Geometry check sheet. Reference: the model listing, model coordinates, mm. Coordinates: 2 decimals unless noted, no trailing zeros. Order: outer loops, then holes, each group sorted by start corner. A loop starts at its lowest first (then second) coordinate and runs counter-clockwise, first axis right, second up. Notation, with made-up numbers: (-5, 57.5) -> (22, 57.5) arc R28 cw to (22, 94.5) -> close; hole circle Ø4 at (78, 7). An arc over 180 degrees is marked (long way). Answer as CSV lines item,"result". Start each with the question number.
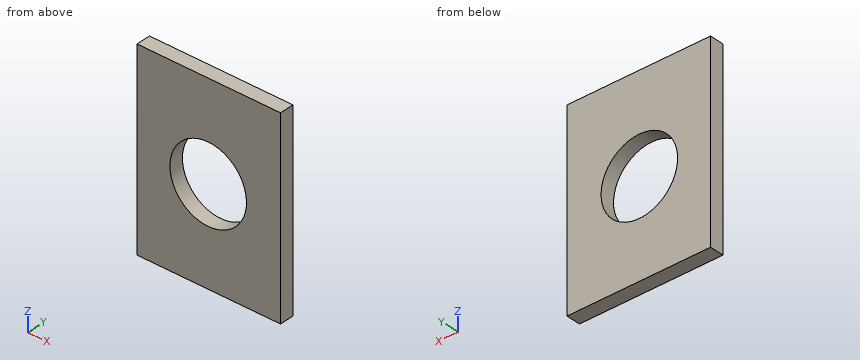
from build123d import *

# Parameters (mm, degrees)
BOSS_EXTRUDE1_DEPTH = 20
BOSS_EXTRUDE2_DEPTH = 1.5
SKETCH3_W           = 10
SKETCH3_H           = 2
BOSS_EXTRUDE3_DEPTH = 100
SKETCH4_R           = 1.55
CUT_EXTRUDE1_DEPTH  = 2
SKETCH5_R           = 4
CUT_EXTRUDE2_DEPTH  = 3
CUT_EXTRUDE3_START  = -2
CUT_EXTRUDE3_DEPTH  = 2
SKETCH7_W           = 92.843167551
SKETCH7_H           = 36.119357845
CUT_EXTRUDE4_DEPTH  = 30
SKETCH8_W           = 90.626752411
SKETCH8_H           = 35.380552798
CUT_EXTRUDE5_DEPTH  = 55
SKETCH10_W          = 29.390209747
SKETCH10_H          = 30.061690813
CUT_EXTRUDE7_DEPTH  = 20
SKETCH11_W          = 23.008025921
SKETCH11_H          = 26.899718038
CUT_EXTRUDE8_DEPTH  = 40


# Read off the part's stored shape, not the designer's step: Boss-Extrude1, Cut-Extrude3
with BuildPart() as part:
    # Boss-Extrude1 outline → Boss-Extrude1 (new body)
    with BuildSketch(Plane(origin=(0, 0, 0), x_dir=(1, 0, 0), z_dir=(0, 1, 0))):
        with BuildLine():
            Line((49.999999852, 30), (4.999999852, 30))
            ThreePointArc((4.999999852, 30), (1.464465946, 31.464466094), (-1.48e-07, 35))
            Line((-1.48e-07, 35), (-1.48e-07, 40))
            Line((-1.48e-07, 40), (-40.000000148, 40))
            Line((-40.000000148, 40), (-40.000000111, 35))
            ThreePointArc((-40.000000111, 35), (-41.464466194, 31.46446612), (-45.000000074, 30.000000037))
            Line((-45.000000074, 30.000000037), (-50.000000148, 30))
            Line((-50.000000148, 30), (-50.000000148, -30))
            Line((-50.000000148, -30), (49.999999852, -30))
            Line((49.999999852, -30), (49.999999852, 30))
        make_face()
        with BuildLine():
            Line((-48.5, 28.5), (-44.999018222, 28.5))
            ThreePointArc((-44.999018222, 28.5), (-40.40345882, 30.40415302), (-38.5, 35))
            Line((-38.5, 35), (-38.5, 38.5))
            Line((-38.5, 38.5), (-1.500000148, 38.5))
            Line((-1.500000148, 38.5), (-1.500000148, 35))
            ThreePointArc((-1.500000148, 35), (0.403805774, 30.403805922), (4.999999852, 28.5))
            Line((4.999999852, 28.5), (48.5, 28.5))
            Line((48.5, 28.5), (48.5, -28.5))
            Line((48.5, -28.5), (-48.5, -28.5))
            Line((-48.5, -28.5), (-48.5, 28.5))
        make_face(mode=Mode.SUBTRACT)
    extrude(amount=BOSS_EXTRUDE1_DEPTH)

    # Sketch2 → Boss-Extrude2 (add)
    with BuildSketch(Plane(origin=(0, 20, 0), x_dir=(1, 0, 0), z_dir=(0, 1, 0))):
        with BuildLine():
            Line((-40.000000148, 40), (-1.48e-07, 40))
            Line((-1.48e-07, 40), (-1.48e-07, 35))
            ThreePointArc((-1.48e-07, 35), (1.464465946, 31.464466094), (4.999999852, 30))
            Line((4.999999852, 30), (49.999999852, 30))
            Line((49.999999852, 30), (49.999999852, -30))
            Line((49.999999852, -30), (-50.000000148, -30))
            Line((-50.000000148, -30), (-50.000000148, 30))
            Line((-50.000000148, 30), (-45.000000074, 30))
            ThreePointArc((-45.000000074, 30), (-41.464466216, 31.46446612), (-40.000000148, 35))
            Line((-40.000000148, 35), (-40.000000148, 40))
        make_face()
    extrude(amount=BOSS_EXTRUDE2_DEPTH)

    # Sketch3 → Boss-Extrude3 (add)
    with BuildSketch(Plane(origin=(49.999999852, 0, 0), x_dir=(0, 0, -1), z_dir=(1, 0, 0))):
        with Locations((35, 1)):
            Rectangle(SKETCH3_W, SKETCH3_H)
        with Locations((-35, 1)):
            Rectangle(SKETCH3_W, SKETCH3_H)
    extrude(amount=-BOSS_EXTRUDE3_DEPTH)

    # Sketch4 → Cut-Extrude1 (cut)
    with BuildSketch(Plane.XZ):
        with Locations(Location((-45, 35, 0), (0, 0, 270))):
            Circle(SKETCH4_R)
        with Locations(Location((45, 35, 0), (0, 0, 270))):
            Circle(SKETCH4_R)
        with Locations(Location((45, -35, 0), (0, 0, 270))):
            Circle(SKETCH4_R)
        with Locations(Location((-45, -35, 0), (0, 0, 270))):
            Circle(SKETCH4_R)
        with Locations(Location((5, 35, 0), (0, 0, 270))):
            Circle(SKETCH4_R)
        with Locations(Location((5, -35, 0), (0, 0, 270))):
            Circle(SKETCH4_R)
    extrude(amount=-CUT_EXTRUDE1_DEPTH, mode=Mode.SUBTRACT)

    # Sketch5 → Cut-Extrude2 (cut)
    with BuildSketch(Plane(origin=(0, 21.5, 0), x_dir=(1, 0, 0), z_dir=(0, 1, 0))):
        with Locations(Location((12.44, -9.95, 0), (0, 0, 270))):
            Circle(SKETCH5_R)
    extrude(amount=-CUT_EXTRUDE2_DEPTH, mode=Mode.SUBTRACT)

    # Cut-Extrude3 outline → Cut-Extrude3 (cut)
    with BuildSketch(Plane(origin=(0, 2, 0), x_dir=(1, 0, 0), z_dir=(0, 1, 0)).offset(CUT_EXTRUDE3_START)):
        with BuildLine():
            Line((-38.5, 38.5), (-38.5, 35))
            ThreePointArc((-38.5, 35), (-39.115846372, 32.238345392), (-40.846688027, 30))
            Line((-40.846688027, 30), (0.84668792, 30))
            ThreePointArc((0.84668792, 30), (-0.884153764, 32.238345383), (-1.500000148, 35))
            Line((-1.500000148, 35), (-1.500000148, 38.5))
            Line((-1.500000148, 38.5), (-38.5, 38.5))
        make_face()
    extrude(amount=CUT_EXTRUDE3_DEPTH, mode=Mode.SUBTRACT)

    # Sketch7 → Cut-Extrude4 (cut)
    with BuildSketch(Plane(origin=(49.999999852, 0, 0), x_dir=(0, 0, -1), z_dir=(1, 0, 0))):
        with Locations((0.287313074, 10.115071794)):
            Rectangle(SKETCH7_W, SKETCH7_H)
    extrude(amount=-CUT_EXTRUDE4_DEPTH, mode=Mode.SUBTRACT)

    # Sketch8 → Cut-Extrude5 (cut)
    with BuildSketch(Plane.ZY.offset(50.000000148)):
        with Locations((-1.067162845, 10.564009403)):
            Rectangle(SKETCH8_W, SKETCH8_H)
    extrude(amount=-CUT_EXTRUDE5_DEPTH, mode=Mode.SUBTRACT)

    # Sketch10 → Cut-Extrude7 (cut)
    with BuildSketch(Plane.XY.offset(40)):
        with Locations((11.70310279, 9.975782262)):
            Rectangle(SKETCH10_W, SKETCH10_H)
    extrude(amount=-CUT_EXTRUDE7_DEPTH, mode=Mode.SUBTRACT)

    # Sketch11 → Cut-Extrude8 (cut)
    with BuildSketch(Plane(origin=(0, 0, -40), x_dir=(-1, 0, 0), z_dir=(0, 0, -1))):
        with Locations((-13.617747202, 10.15531134)):
            Rectangle(SKETCH11_W, SKETCH11_H)
    extrude(amount=-CUT_EXTRUDE8_DEPTH, mode=Mode.SUBTRACT)


solid = part.part
Q1. Thickness scan on L1, parallel to X at y = 20.9, z = 9.95; L2, parallel to Z at x = 9.75, y = 20.95; L3, parallel to Z at x = 9, y = 21.1. Record the ranges inside material, lowest first.
Q2. Sectioned sample at B-B, the plane z = 9.95. Record the cut outline in (x, y), then the cut area to 3 significant figures.
Q3. Go/stop test with flat-tipped pins: pin 1 Ø8 at (x, z) = (14, 9.5) entering from +Y; pin 2 Ø6.5 at (x, z) = (12.44, 9.95) entering from -Y. Record where each tip stops, or that it passes through.
Q4. Sectioned sample at A-A, the plane x = 12.44. Record the cut outline in (y, z), then the cut area to 3 significant figures.
Q5. Sectioned sample at C-C, the plane y = 21.1. Record the cut outline in (x, z).
Geometry results:
1,L1,"x = 5 to 8.44, 16.44 to 20"
1,L2,"z = 0 to 6.99, 12.91 to 20"
1,L3,"z = 0 to 7.91, 11.99 to 20"
2,outline,"(5, 20) -> (8.44, 20) -> (8.44, 21.5) -> (5, 21.5) -> close; (16.44, 20) -> (20, 20) -> (20, 21.5) -> (16.44, 21.5) -> close"
2,area,"10.5 mm^2"
3,pin 1,"stops at y = 21.5"
3,pin 2,"passes through"
4,outline,"(20, 0) -> (21.5, 0) -> (21.5, 5.95) -> (20, 5.95) -> close; (20, 13.95) -> (21.5, 13.95) -> (21.5, 20) -> (20, 20) -> close"
4,area,"18.0 mm^2"
5,outline,"(5, 0) -> (20, 0) -> (20, 20) -> (5, 20) -> close; hole circle Ø8 at (12.44, 9.95)"
